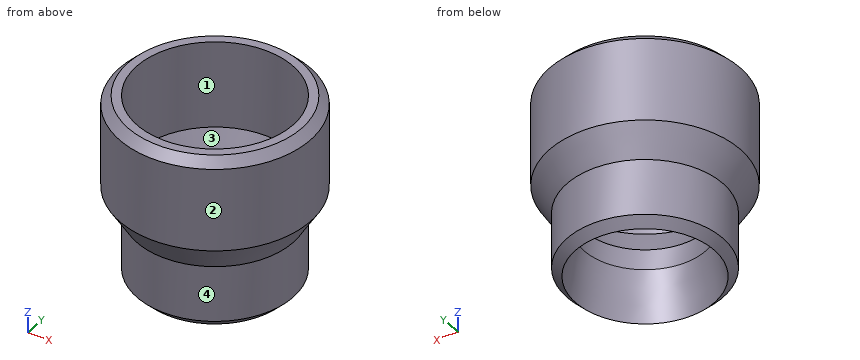
from build123d import *

# Parameters (mm, degrees)
F2_SIZE2 = 1
F2_SIZE  = 1
F3_SIZE2 = 0.99999
F3_SIZE  = 5.671272


# Not quite as in the source:
# - a fillet or chamfer is up to 0.001 mm smaller than in the source, because OpenCascade refuses the exact size


with BuildPart() as f1:
    # F0 (on Front) → F1 (revolve)
    with BuildSketch(Plane.XZ):
        Polygon((-9, 0), (-9, 10), (-11, 10), (-11, -0.5671153529), (-9, -3.8101770668), (-9, -11.2430617139), (-7, -11.2430617139), (-7, -3.2430617139), align=None)
    revolve(axis=Axis((0, 0, -1.2268370084), (0, 0, -1)))

    # F2
    f2_edges = [f1.edges().sort_by_distance(p)[0] for p in [
        (9, 0, -11.243062),
        (11, 0, 10),
    ]]
    chamfer(f2_edges, length=F2_SIZE, length2=F2_SIZE2)

    # F3 (size 5.6712818196 and 1 in the source; OpenCascade refuses exactly that, so slightly less here)
    f3_edges = [f1.edges().sort_by_distance(p)[0] for p in [
        (7, 0, -11.243062),
    ]]
    f3_side = f1.faces().sort_by_distance((7, 0, -7.243062))[0]
    chamfer(f3_edges, length=F3_SIZE, length2=F3_SIZE2, reference=f3_side)


solid = f1.part
Model file for the job. Use its own axes, mm. Face numbers are marked on the shaded views. A direction names the side the tool comes from. Coordinates: 2 decimals unless noted, no trailing zeros. Order: outer loops, then holes, each group sorted by start corner. A loop starts at its lowest first (then second) coordinate and runs counter-clockwise, first axis right, second up. Notation, with made-up numbers: (82, 73) -> (97, 73) arc R22 ccw to (97, 106) -> close; hole circle Ø4 at (4.5, 56). An arc over 180 degrees is marked (long way). Return JSON: item names as keys, results as strings. Group by question number.
Item 1: Pull direction Y, two halves, no side cores. Call the marked faces 1 and 2: pulls with the +Y half, pulls with the -Y half, needs draft (parallel to the pull), parting line crosses it, or undercut.
Item 2: Tool access for the marked faces 3 and 4: list every direction of +Z, -Z, +X, -X, +Y, -Y with a clear straight run to the whole face (end or side of a thin tool).
Item 3: Flat gauge pins, fed straight in: P1, Ø1.5, axis at x = 3.5, z = 0, coming from the -Y side; P2, Ø5, axis at y = 5.5, z = -9, coming from the -X side; P3, Ø12, axis at y = 8, z = 6, coming from the +X side. Where does each tip first touch, or does it go through?
Item 4: Saw through at D-D on z = -6.5. Write the cut outline in (x, y).
Item 5: Saw through at C-C on z = 8. Write the cut outline in (x, y), then the cut area to 3 significant figures.
Item 6: Wall check: line 1 along Y through (x, z) = (0, 5.5); line 2 along Y through (x, z) = (0, -4.4); line 3 along X through (y, z) = (5.75, -7). Give the ranges that are in metal, low to high. Write a range as [from, to].
Values found:
{
 "1": {"face 1": "undercut", "face 2": "parting line crosses it"},
 "2": {"face 3": "+Z", "face 4": "-Z"},
 "3": {"P1": "stops at y = -10.65", "P2": "stops at x = -8.49", "P3": "stops at x = 10.82"},
 "4": {"outline": "circle Ø18 at (0, 0); hole circle Ø14.33 at (0, 0)"},
 "5": {"outline": "circle Ø22 at (0, 0); hole circle Ø18 at (0, 0)", "area": "126 mm2"},
 "6": {"line 1": "y = [-11, -9], [9, 11]", "line 2": "y = [-9, -7], [7, 9]", "line 3": "x = [-6.92, -4.42], [4.42, 6.92]"}
}
